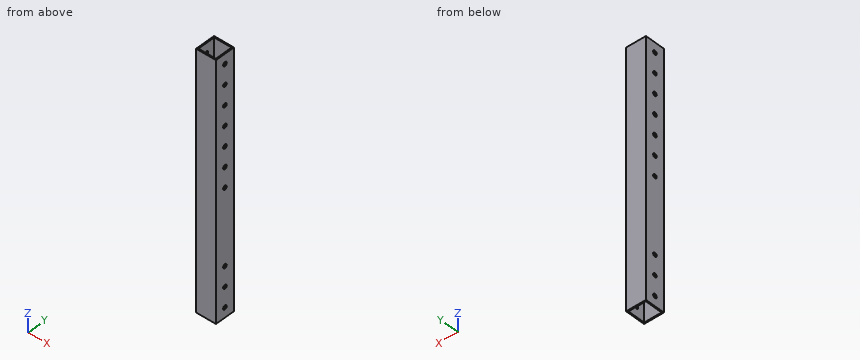
Autodesk Inventor part; units mm, degrees
ref_plane "YZ Plane" through (0, 0, 0) normal (1, 0, 0) x (0, 1, 0)
ref_plane "XZ Plane" through (0, 0, 0) normal (0, 1, 0) x (-1, 0, 0)
ref_plane "XY Plane" through (0, 0, 0) normal (0, 0, 1) x (1, 0, 0)
sketch "Sketch1" plane through (0, 0, 0) normal (0, 0, 1) x (1, 0, 0)
  line L0 (-12.7, -12.7) -> (-12.7, 12.7)
  line L1 (-12.7, 12.7) -> (12.7, 12.7)
  line L2 (12.7, 12.7) -> (12.7, -12.7)
  line L3 (12.7, -12.7) -> (-12.7, -12.7)
  line L4 (-12.7, -12.7) -> (12.7, 12.7) construction
  line L5 (-12.7, 12.7) -> (12.7, -12.7) construction
  line L6 (11.1125, 11.1125) -> (-11.1125, 11.1125)
  line L7 (-11.1125, 11.1125) -> (-11.1125, -11.1125)
  line L8 (-11.1125, -11.1125) -> (11.1125, -11.1125)
  line L9 (11.1125, -11.1125) -> (11.1125, 11.1125)
  point P0 (0, 0)
  dimension "d0" = 25.4
  dimension "d1" = 25.4
  dimension "d2" = 1.5875
extrude "Extrusion1" add sketch "Sketch1" along normal blind 609.6
sketch "Sketch2" plane through (12.7, -12.7, 0) normal (1, 0, 0) x (0, 0, -1)
  line L0 (0, 0) -> (0, 25.4)
  line L1 (0, 25.4) -> (-609.6, 25.4)
  line L2 (-609.6, 0) -> (-609.6, 25.4)
  line L3 (0, 0) -> (-609.6, 0)
  circle A0 centre (-596.9, 12.7) radius 2.5781
  circle A1 centre (-571.5, 12.7) radius 2.5781
  circle A2 centre (-546.1, 12.7) radius 2.5781
  line L4 (-304.8, 0) -> (-304.8, 25.4) construction
  circle A3 centre (-12.7, 12.7) radius 2.5781
  circle A4 centre (-38.1, 12.7) radius 2.5781
  circle A5 centre (-63.5, 12.7) radius 2.5781
  point P0 (0, 12.7)
  dimension "d5" = 5.1562
  dimension "d7" = 12.7
  dimension "d8" = 25.4
  dimension "d9" = 25.4
extrude "Extrusion2" cut sketch "Sketch2" against normal through all contours A0 | A1 | A2 | A3 | A4 | A5
sketch "Sketch5" plane through (-12.7, 12.7, 0) normal (0, 1, 0) x (1, 0, 0)
  line L0 (25.4, 0) -> (25.4, -609.6)
  line L1 (25.4, 0) -> (25.4, -223.7994)
  line L2 (25.4, -223.7994) -> (-0.9, -223.7994)
  line L3 (-0.9, -223.7994) -> (-0.9, -681.5571)
  line L4 (-0.9, -681.5571) -> (85.6151, -690.7866)
  line L5 (85.6151, -690.7866) -> (25.4, -223.7994)
  point P0 (12.7, 0)
  dimension "d15" = 223.7994
extrude "Extrusion4" cut sketch "Sketch5" against normal blind 101.6
sketch "Sketch6" plane through (12.7, -12.7, 0) normal (1, 0, 0) x (0, 0, -1)
  line L0 (-223.7994, 1.5875) -> (-223.7994, 23.8125)
  line L1 (-223.7994, 12.7) -> (-211.0994, 12.7)
  circle A0 centre (-211.0994, 12.7) radius 2.5781
  line L2 (-211.0994, 12.7) -> (-185.6994, 12.7)
  circle A1 centre (-185.6994, 12.7) radius 2.5781
  line L3 (-185.6994, 12.7) -> (-160.2994, 12.7)
  circle A2 centre (-160.2994, 12.7) radius 2.5781
  point P0 (0, 12.7)
  dimension "d18" = 12.7
  dimension "d19" = 5.1562
  dimension "d20" = 25.4
  dimension "d21" = 5.1562
  dimension "d22" = 25.4
  dimension "d23" = 5.1562
extrude "Extrusion5" cut sketch "Sketch6" against normal blind 50.8
sketch "Sketch7" plane through (-12.7, 12.7, 223.7994) normal (0, 0, 1) x (1, 0, 0)
  line L0 (0, -25.4) -> (0, 0)
  line L1 (25.4, -25.4) -> (0, -25.4)
  line L2 (25.4, 0) -> (25.4, -25.4)
  line L3 (0, 0) -> (25.4, 0)
  line L4 (23.8125, -1.5875) -> (1.5875, -1.5875)
  line L5 (23.8125, -23.8125) -> (23.8125, -1.5875)
  line L6 (1.5875, -23.8125) -> (23.8125, -23.8125)
  line L7 (1.5875, -1.5875) -> (1.5875, -23.8125)
  point P0 (12.7, -12.7)
extrude "Extrusion6" add sketch "Sketch7" along normal blind 127
sketch "Sketch8" plane through (12.7, -12.7, 0) normal (1, 0, 0) x (0, 0, -1)
  circle A0 centre (-211.0994, 12.7) radius 2.5781
  line L0 (-211.0994, 12.7) -> (-236.4994, 12.7)
  line L1 (-236.4994, 12.7) -> (-261.8994, 12.7)
  circle A1 centre (-236.4994, 12.7) radius 2.5781
  circle A2 centre (-261.8994, 12.7) radius 2.5781
  line L2 (-350.7994, 25.4) -> (-350.7994, 0)
  line L3 (-350.7994, 12.7) -> (-338.0994, 12.7)
  line L4 (-338.0994, 12.7) -> (-312.6994, 12.7)
  line L5 (-312.6994, 12.7) -> (-287.2994, 12.7)
  circle A3 centre (-287.2994, 12.7) radius 2.5781
  circle A4 centre (-338.0994, 12.7) radius 2.5781
  circle A5 centre (-312.6994, 12.7) radius 2.5781
  point P0 (0, 12.7)
  dimension "d28" = 25.4
  dimension "d29" = 25.4
  dimension "d30" = 5.1562
  dimension "d31" = 5.1562
  dimension "d32" = 12.7
  dimension "d33" = 25.4
  dimension "d34" = 25.4
  dimension "d35" = 5.1562
  dimension "d36" = 5.1562
  dimension "d37" = 5.1562
extrude "Extrusion7" cut sketch "Sketch8" against normal blind 92.075 contours A2 | A1 L1 L0 | L0 L1 A1 | A4 L4 L3 | A3 | A5 L5 L4 | L4 L5 A5 | L3 L4 A4
sketch "Sketch9" plane through (0, 0, 0) normal (0, 0, -1) x (-1, 0, 0)
  line L0 (-12.7, -12.7) -> (-12.7, 12.7)
  line L1 (12.7, -12.7) -> (-12.7, -12.7)
  line L2 (12.7, 12.7) -> (12.7, -12.7)
  line L3 (-12.7, 12.7) -> (12.7, 12.7)
  line L4 (-11.1125, 11.1125) -> (-11.1125, -11.1125)
  line L5 (11.1125, 11.1125) -> (-11.1125, 11.1125)
  line L6 (11.1125, -11.1125) -> (11.1125, 11.1125)
  line L7 (-11.1125, -11.1125) -> (11.1125, -11.1125)
  point P0 (0, 0)
extrude "Extrusion8" add sketch "Sketch9" along normal blind 152.4
sketch "Sketch10" plane through (12.7, -12.7, 350.7994) normal (1, 0, 0) x (0, 0, -1)
  line L0 (503.1994, 25.4) -> (503.1994, 0)
  line L1 (503.1994, 12.7) -> (490.4994, 12.7)
  line L2 (490.4994, 12.7) -> (465.0994, 12.7)
  line L3 (465.0994, 12.7) -> (439.6994, 12.7)
  circle A0 centre (439.6994, 12.7) radius 2.5781
  circle A1 centre (465.0994, 12.7) radius 2.5781
  circle A2 centre (490.4994, 12.7) radius 2.5781
  point P0 (350.7994, 12.7)
  dimension "d42" = 12.7
  dimension "d43" = 25.4
  dimension "d44" = 25.4
  dimension "d45" = 5.1562
  dimension "d46" = 5.1562
  dimension "d47" = 5.1562
extrude "Extrusion9" cut sketch "Sketch10" against normal blind 123.825
sketch "Sketch11" plane through (0, 0, -152.4) normal (0, 0, -1) x (-1, 0, 0)
  line L0 (12.7, -12.7) -> (12.7, 12.7)
  line L1 (12.7, 12.7) -> (-12.7, 12.7)
  line L2 (-12.7, 12.7) -> (-12.7, -12.7)
  line L3 (-12.7, -12.7) -> (12.7, -12.7)
  line L4 (-11.1125, 11.1125) -> (11.1125, 11.1125)
  line L5 (11.1125, 11.1125) -> (11.1125, -11.1125)
  line L6 (11.1125, -11.1125) -> (-11.1125, -11.1125)
  line L7 (-11.1125, -11.1125) -> (-11.1125, 11.1125)
  point P0 (0, 0)
extrude "Extrusion10" cut sketch "Sketch11" against normal blind 152.4
sketch "Sketch12" plane through (-12.7, 12.7, 350.7994) normal (0, 0, 1) x (1, 0, 0)
  line L0 (25.4, -25.4) -> (25.4, 0)
  line L1 (25.4, 0) -> (0, 0)
  line L2 (0, 0) -> (0, -25.4)
  line L3 (0, -25.4) -> (25.4, -25.4)
  line L4 (23.8125, -1.5875) -> (23.8125, -23.8125)
  line L5 (23.8125, -23.8125) -> (1.5875, -23.8125)
  line L6 (1.5875, -23.8125) -> (1.5875, -1.5875)
  line L7 (1.5875, -1.5875) -> (23.8125, -1.5875)
  point P0 (12.7, -12.7)
extrude "Extrusion11" add sketch "Sketch12" along normal blind 63.5
sketch "Sketch13" plane through (12.7, -12.7, 0) normal (1, 0, 0) x (0, 0, -1)
  circle A0 centre (-338.0994, 12.7) radius 2.5781
  line L0 (-338.0994, 12.7) -> (-363.4994, 12.7)
  line L1 (-363.4994, 12.7) -> (-388.8994, 12.7)
  line L2 (-388.8994, 12.7) -> (-414.2994, 12.7)
  circle A1 centre (-363.4994, 12.7) radius 2.5781
  circle A2 centre (-388.8994, 12.7) radius 2.5781
  circle A3 centre (-414.2994, 12.7) radius 2.5781
  point P0 (0, 12.7)
  dimension "d54" = 25.4
  dimension "d55" = 25.4
  dimension "d58" = 25.4
  dimension "d59" = 5.1562
  dimension "d60" = 5.1562
  dimension "d61" = 5.1562
sketch "Sketch14" plane through (-12.7, 12.7, 414.2994) normal (0, 0, 1) x (1, 0, 0)
  line L0 (25.4, 0) -> (0, 0)
  line L1 (0, 0) -> (0, -25.4)
  line L2 (0, -25.4) -> (25.4, -25.4)
  line L3 (25.4, -25.4) -> (25.4, 0)
  line L4 (23.8125, -1.5875) -> (23.8125, -23.8125)
  line L5 (23.8125, -23.8125) -> (1.5875, -23.8125)
  line L6 (1.5875, -23.8125) -> (1.5875, -1.5875)
  line L7 (1.5875, -1.5875) -> (23.8125, -1.5875)
  point P0 (12.7, -12.7)
extrude "Extrusion12" add sketch "Sketch14" along normal blind 12.7
extrude "Extrusion13" cut sketch "Sketch13" against normal blind 47.625 contours A3 | A2 L2 L1 | L1 L2 A2 | A1 L1 L0 | L0 L1 A1
sketch "Sketch15" plane through (12.7, -12.7, 0) normal (1, 0, 0) x (0, 0, -1)
  circle A0 centre (-363.4994, 12.7) radius 2.5781
  line L0 (-363.4994, 12.7) -> (-376.1994, 12.7)
  line L1 (-376.1994, 12.7) -> (-376.1994, 25.4)
  line L2 (0, 25.4) -> (-426.9994, 25.4)
  line L3 (-376.1994, 12.7) -> (-376.1994, -0.0996)
  line L4 (-376.1994, -0.0996) -> (-376.1994, -3.0916)
  line L5 (-376.1994, -3.0916) -> (-480.1709, -3.0916)
  line L6 (-480.1709, -3.0916) -> (-483.3081, 73.6134)
  line L7 (-483.3081, 73.6134) -> (-376.1994, 25.4)
  point P0 (0, 12.7)
  dimension "d64" = 12.7
extrude "Extrusion14" cut sketch "Sketch15" against normal blind 47.625 contours L3 L4 L5 L6 L7 L1
sketch "Sketch17" plane through (12.7, -12.7, 0) normal (1, 0, 0) x (0, 0, -1)
  circle A0 centre (-312.6994, 12.7) radius 2.5781
  line L0 (-312.6994, 12.7) -> (-325.3994, 12.7)
  line L1 (0, 25.4) -> (-376.1994, 25.4)
  line L2 (-325.3994, 25.4) -> (-387.8769, 25.4)
  line L3 (-387.8769, 25.4) -> (-387.8769, -7.9808)
  line L4 (-387.8769, -7.9808) -> (-325.3994, -7.9808)
  line L5 (-325.3994, -7.9808) -> (-325.3994, 25.4)
  point P0 (0, 12.7)
  dimension "d67" = 12.7
extrude "Extrusion15" cut sketch "Sketch17" against normal blind 112.7125 contours L5 L4 L3 L2 L1
equation "\"d1\" = d0"
properties part number "24in long 1in square tube"
Work out the finished part from the listing and answer in its coordinate system (mm). Coordinates: 2 decimals unless noted, no trailing zeros. Order: outer loops, then holes, each group sorted by start corner. A loop starts at its lowest first (then second) coordinate and runs counter-clockwise, first axis right, second up. Notation, with made-up numbers: (77.25, 13) - (107.25, 13) arc R35 cw to (107.25, 47) - close; hole circle Ø9 at (-3, -0.75). An arc over 180 degrees is marked (long way). Answer as a JSON object with one key per item and string values.
1. Each of these flat-tipped pins is pushed along its axis until it touches: P1, Ø6.5, axis at y = 0, z = 211.1, coming from the -X side; P2, Ø3, axis at y = 0, z = 12.7, coming from the +X side (3 decimals). Where does it stop, or does it pass through?
Output values:
{"P1": "stops at x = -12.7", "P2": "passes through"}
2. Find section A-A on x = -1.5. Determine the outline of the cut face in (y, z), plus the area to 3 significant figures.
Output values:
{"outline": "(-12.7, 0) - (-11.11, 0) - (-11.11, 325.4) - (-12.7, 325.4) - close; (11.11, 0) - (12.7, 0) - (12.7, 325.4) - (11.11, 325.4) - close", "area": "1,030 mm²"}
3. Find section C-C on z = 276. Determine the outline of the cut face in (x, y).
Output values:
{"outline": "(-12.7, -12.7) - (12.7, -12.7) - (12.7, 12.7) - (-12.7, 12.7) - close; hole (-11.11, -11.11) - (11.11, -11.11) - (11.11, 11.11) - (-11.11, 11.11) - close"}
4. Consider line 1 (Y direction, x = -3.25, z = 217); line 2 (Y direction, x = -11.7, z = 63.5). Determine where each line is inside the solid, lowest interval first.
Output values:
{"line 1": "y = -12.7 to -11.11, 11.11 to 12.7", "line 2": "y = -12.7 to -2.58, 2.58 to 12.7"}
